Autodesk Fusion 360 part; units mm, degrees
sketch "Sketch1" plane through (0, 0, 0) normal (0, 0, 1) x (1, 0, 0)
  circle A0 centre (0, 0) radius 1.75
  circle A1 centre (0, 0) radius 5
  circle A2 centre (0, 0) radius 3.5
  circle A3 centre (-26, 0) radius 4
  line L0 (-25.9137, 3.9991) -> (-3.0012, 3.9991)
  line L1 (-25.9137, -3.9991) -> (-3.0012, -3.9991)
  dimension "d1" = 3.5
  dimension "d2" = 10
  dimension "d3" = 7
  dimension "d4" = 8
extrude "Extrude1" add sketch "Sketch1" against normal blind 18 contours A1 makes body 1
extrude "Extrude2" add sketch "Sketch1" along normal blind -12 and the other way blind 18 contours A2 bodies 1
extrude "Extrude3" add sketch "Sketch1" against normal blind 6 contours A1 A3 L0 L1 | A3 bodies 1
sketch "Sketch2" plane through (0, 0, 0) normal (1, 0, 0) x (0, 1, 0)
  line L0 (-10, 7) -> (14, 7)
  line L1 (14, 7) -> (14, 2)
  line L2 (14, 2) -> (-10, 2)
  line L3 (-10, 2) -> (-10, 7)
  line L4 (14, 7) -> (19, 7)
  line L5 (19, 7) -> (19, -9)
  line L6 (19, -9) -> (14, -9)
  line L7 (14, -9) -> (14, 7)
  line L8 (19, -9) -> (27.5, -9)
  line L9 (27.5, -9) -> (27.5, -3)
  line L10 (27.5, -3) -> (19, -3)
  line L11 (19, -3) -> (19, -9)
extrude "Extrude4" add sketch "Sketch2" against normal blind 6 separate body makes body 2
sketch "Sketch3" plane through (0, 0, -3) normal (0, 0, 1) x (-1, 0, 0)
  line L0 (0, -19) -> (0, -27.5)
  line L1 (0, -27.5) -> (6, -27.5)
  line L2 (6, -27.5) -> (6, -19)
  line L3 (6, -19) -> (0, -19)
  circle A0 centre (3, -23.25) radius 1.75
  dimension "d15" = 3.5
extrude "Extrude5" cut sketch "Sketch3" against normal blind 15 contours A0 bodies 2
fillet "Fillet1" radius 2.5 2 edges at (-6, -10, 4.5) (0, -10, 4.5) on bodies 2
hidden bodies 1
Input: part model. Units: mm. Frame: model coordinates. A direction names the side the tool comes from. Coordinates: 2 decimals unless noted, no trailing zeros. Write each loop counter-clockwise with the first axis right and the second up, starting at its lowest first coordinate (ties: lowest second). Pieces come first, ordered by that corner, then holes.
1) Section D-D on z = 4.75. Output: boundary loops of the cut face in (x, y).
2) Section A-A on x = -3. Output: boundary loops of the cut face in (y, z).
3) Section C-C on x = -0.5. Output: boundary loops of the cut face in (y, z), and give its area (3 significant figures).
4) Set-up query: faces 5 (the flat face through (-3, 21, -3)), 6 (the flat face through (-3, 14, -4)), 7 (the flat face through (-3, 4, 7)). Return all of +Z, -Z, +X, -X, +Y, -Y with unobstructed straight access to the full face (end or side cutting, diameter ignored); none if empty.
5) Material intervals for line 1 along Y through (x, z) = (-3, -5.5); line 2 along X through (y, z) = (23.25, -6.05); line 3 along Z through (x, y) = (-2.05, -4), sorted ascending.
6) Mould query, pull axis Y, two halves, no side actions, for faces 1 (the cylindrical face through (-2.772, 21.515, -5.958)), 2 (the cylindrical face through (-0.752, -9.287, 4.535)), 3 (the flat face through (0, 10, 3)), 4 (the flat face through (-3, 19, 2)). Classes: pulls with the +Y half, pulls with the -Y half, needs draft (parallel to the pull), parting line crosses it, or undercut.
7) Section B-B on y = 23.25. Output: boundary loops of the cut face in (x, z).
8) Pin query (flat end, axial travel): pin 1 Ø1.8 at (x, z) = (-1.5, 2.5) entering from +Y; pin 2 Ø1.5 at (x, y) = (-1, 6) entering from -Z; pin 3 Ø1 at (x, z) = (-3, -4) entering from -Y. Return the tip coordinate at first contact, or that it passes through.
Check result:
1. outline: (-6, -7.5) arc R2.5 ccw to (-3.5, -10) - (-2.5, -10) arc R2.5 ccw to (0, -7.5) - (0, 19) - (-6, 19) - close
2. outline: (-10, 2) - (14, 2) - (14, -9) - (21.5, -9) - (21.5, -3) - (19, -3) - (19, 7) - (-10, 7) - close; (25, -9) - (27.5, -9) - (27.5, -3) - (25, -3) - close
3. outline: (-9, 2) - (14, 2) - (14, -9) - (27.5, -9) - (27.5, -3) - (19, -3) - (19, 7) - (-9, 7) - close
3. area: 246 mm2
4. face 5: +Z, +X, -X, +Y
4. face 6: -Z, +X, -X, -Y
4. face 7: +Z, +X, -X, +Y, -Y
5. line 1: y = 14 to 21.5, 25 to 27.5
5. line 2: x = -6 to -4.75, -1.25 to 0
5. line 3: z = 2 to 7
6. face 1: undercut
6. face 2: pulls with the -Y half
6. face 3: needs draft
6. face 4: pulls with the +Y half
7. outline: (-6, -9) - (-4.75, -9) - (-4.75, -3) - (-6, -3) - close; (-1.25, -9) - (0, -9) - (0, -3) - (-1.25, -3) - close
8. pin 1: stops at y = 19
8. pin 2: stops at z = 2
8. pin 3: stops at y = 14
